Read the model definition and answer for the solid it produces. Units are mm, in the model's axes. A direction names the side the tool comes from. Coordinates: 2 decimals unless noted, no trailing zeros. Loops run counter-clockwise (first coordinate to the right, second up) from the corner with the lowest first, then second, coordinate; pieces in that order, holes last. Notation, with made-up numbers: (44.25, 8) - (50.25, 8) arc R22 ccw to (50.25, 24) - close; hole circle Ø9 at (-26, 61). An arc over 180 degrees is marked (long way). Use one line per item in the form item = value.
from build123d import *

# Parameters (mm, degrees)
SKETCH1_R           = 1.75
SKETCH1_R_2         = 0.75
BOSS_EXTRUDE1_DEPTH = 1.85
CUT_EXTRUDE1_DEPTH  = 0.85


with BuildPart() as part:
    # Sketch1 → Boss-Extrude1 (new body, symmetric)
    with BuildSketch(Plane.XY):
        with BuildLine():
            Line((-2.248747058, 9.975077763), (-2.450586667, 3.929529668))
            ThreePointArc((-2.450586667, 3.929529668), (-2.626439392, 2.771809131), (-3.066742144, 1.686740235))
            ThreePointArc((-3.066742144, 1.686740235), (-3.115718571, -1.594458461), (-0.425746012, -3.474009259))
            ThreePointArc((-0.425746012, -3.474009259), (0.794490836, -3.783194285), (1.898835448, -4.387343542))
            Line((1.898835448, -4.387343542), (3.849546842, -5.800104619))
            ThreePointArc((3.849546842, -5.800104619), (6.502194953, -5.474619694), (6.371070446, -2.805296035))
            Line((6.371070446, -2.805296035), (5.994743374, -2.438319573))
            ThreePointArc((5.994743374, -2.438319573), (5.753103265, -2.154083372), (5.568455785, -1.829914483))
            ThreePointArc((5.568455785, -1.829914483), (3.806333847, 2.668506691), (2.511577358, 7.323017665))
            ThreePointArc((2.511577358, 7.323017665), (2.35023388, 8.243248269), (2.275474866, 9.174520072))
            Line((2.275474866, 9.174520072), (2.248747058, 9.975077763))
            ThreePointArc((2.248747058, 9.975077763), (0, 12.15), (-2.248747058, 9.975077763))
        make_face()
        Circle(SKETCH1_R, mode=Mode.SUBTRACT)
        with Locations((0, 9.9)):
            Circle(SKETCH1_R_2, mode=Mode.SUBTRACT)
        with Locations((5.000791037, -4.210490349)):
            Circle(SKETCH1_R_2, mode=Mode.SUBTRACT)
    extrude(amount=BOSS_EXTRUDE1_DEPTH, both=True)

    # Sketch2 → Cut-Extrude1 (cut, symmetric)
    with BuildSketch(Plane.XY):
        Polygon((1.704938045, -6.98647295), (4.176020114, 1.603907731), (8.214802736, -2.706528486), (6.17955487, -9.771778434), align=None)
        Polygon((-2.39415597, 5.619755358), (2.320198625, 8.506541147), (8.539776122, 16.638706119), (-7.891989788, 11.77086667), align=None)
    extrude(amount=CUT_EXTRUDE1_DEPTH, both=True, mode=Mode.SUBTRACT)


solid = part.part
Item 1: The part is cut by section C-C on x = 0. Give the vertices of the cut face in (y, z), plus the area to 3 significant figures.
Results below:
outline = (-3.54, -1.85) - (-1.75, -1.85) - (-1.75, 1.85) - (-3.54, 1.85) - close; (1.75, -1.85) - (9.15, -1.85) - (9.15, -0.85) - (7.09, -0.85) - (7.09, 0.85) - (9.15, 0.85) - (9.15, 1.85) - (1.75, 1.85) - close; (10.65, -1.85) - (12.15, -1.85) - (12.15, -0.85) - (10.65, -0.85) - close; (10.65, 0.85) - (12.15, 0.85) - (12.15, 1.85) - (10.65, 1.85) - close
area = 33.5 mm²
Item 2: The part is cut by section A-A on z = -0.5. Give the vertices of the cut face in (x, y).
Results below:
outline = (-3.07, 1.69) arc R3.5 ccw to (-0.43, -3.47) arc R5 cw to (1.9, -4.39) - (2.36, -4.72) - (4.18, 1.6) arc R47.37 cw to (2.51, 7.32) arc R10 cw to (2.32, 8.51) - (-2.39, 5.62) - (-2.45, 3.93) arc R5 cw to start; hole circle Ø3.5 at (0, 0)
Item 3: The part is cut by section B-B on y = 0. Give the vertices of the cut face in (x, z), plus the area to 3 significant figures.
Results below:
outline = (-3.5, -1.85) - (-1.75, -1.85) - (-1.75, 1.85) - (-3.5, 1.85) - close; (1.75, -1.85) - (4.79, -1.85) - (4.79, -0.85) - (3.71, -0.85) - (3.71, 0.85) - (4.79, 0.85) - (4.79, 1.85) - (1.75, 1.85) - close
area = 15.9 mm²
Item 4: Each of these flat-tipped pins is pushed along its axis until it touches: P1, Ø1.4, axis at x = 0, y = 9.9, coming from the -Z side; P2, Ø1.5, axis at x = -0.5, z = 1, coming from the -Y side. Where does it stop, or does it pass through?
Results below:
P1 = through
P2 = -3.6
Item 5: The part is cut by section D-D on z = 1.5. Give the vertices of the cut face in (x, y), plus the area to 3 significant figures.
Results below:
outline = (-3.07, 1.69) arc R3.5 ccw to (-0.43, -3.47) arc R5 cw to (1.9, -4.39) - (3.85, -5.8) arc R1.96 ccw to (6.37, -2.81) - (5.99, -2.44) arc R2 cw to (5.57, -1.83) arc R47.37 cw to (2.51, 7.32) arc R10 cw to (2.28, 9.17) - (2.25, 9.98) arc R2.25 ccw to (-2.25, 9.98) - (-2.45, 3.93) arc R5 cw to start; hole circle Ø3.5 at (0, 0); hole circle Ø1.5 at (0, 9.9); hole circle Ø1.5 at (5, -4.21)
area = 93.1 mm²
Item 6: Which of the six approach directions +Z, -Z, +X, -X, +Y, -Y give full straight-line access (tool end or side, diameter ignored) to faces 4 (the flat face through (-1, 9, -0.85)), 5 (the cylindrical face through (2.38, 8.02, 0.03))?
Results below:
face_4 = -X, +Y
face_5 = +Z, -Z, +X, +Y
Item 7: Find the intervals of material crossed by L1, parallel to Y at x = 0.25, z = 1.4; L2, parallel to Z at x = 3, y = -4; L3, parallel to X at y = 9.9, z = 1.45, in increasing order.
Results below:
L1 = -3.6 to -1.73, 1.73 to 9.19, 10.61 to 12.14
L2 = -1.85 to -0.85, 0.85 to 1.85
L3 = -2.25 to -0.75, 0.75 to 2.25
Item 8: For a pull along X with two mould halves and no side action, classify faces 1 (the cylindrical face through (6.475, -5.506, 1.357)), 2 (the flat face through (5, -3, 0.85)), 3 (the cylindrical face through (4.41, -4.67, -1.36)) as +X half, -X half, draft (parallel to the pull), parting line (faces both ways), or undercut.
Results below:
face_1 = parting line
face_2 = draft
face_3 = undercut
